Read the model definition and answer for the solid it produces. Units are mm, in the model's axes. A direction names the side the tool comes from. Coordinates: 2 decimals unless noted, no trailing zeros. Order: outer loops, then holes, each group sorted by start corner. A loop starts at its lowest first (then second) coordinate and runs counter-clockwise, first axis right, second up. Notation, with made-up numbers: (63.25, 75.5) -> (104.25, 75.5) arc R16 ccw to (104.25, 104.5) -> close; hole circle Ø11 at (44.25, -31.5). An arc over 180 degrees is marked (long way). Answer as a JSON object with one key per item and string values. Group by question number.
1) A tool of negligible diameter and unlimited length cuts with its end or side. For faces 5 (the flat face through (-65.936, 9, 25)), 6 (the flat face through (-62, 3.499, 28)), 7 (the flat face through (-68, 11.699, 28)), from which of +Z, -Z, +X, -X, +Y, -Y can it reach the whole face along a straight path? Write none if from no direction.
2) Consider L1, parallel to Y at x = -61.75, z = 22; L2, parallel to X at y = 9.75, z = 46.5; L3, parallel to Z at x = -64.75, y = 9. Determine where each line is inside the solid, lowest interval first.
3) Section B-B on x = -60.75 is taken. Determine the outline of the cut face in (y, z).
4) Section A-A on z = 28 is taken. Determine the outline of the cut face in (x, y).
5) Section C-C on y = 10.5 is taken. Determine the outline of the cut face in (x, z).
6) Given pin 1 (6 mm diameter, centred on y = 8.7, z = 28, fed in from +X); pin 2 (1.5 mm diameter, centred on y = 13.5, z = 15.5, fed in from -X); pin 3 (3 mm diameter, centred on y = 10, z = 34.5, fed in from +X), each flat-ended and moving along its own axis, determine where each tip first touches the part or whether it passes through.
7) Section D-D on z = 52.5 is taken. Determine the outline of the cut face in (x, y), and give its area (3 significant figures).
8) Determine the mould class of faces 1 (the flat face through (-65, 9, 0)), 2 (the cylindrical face through (-67.204, 7.355, 30.108)), 3 (the flat face through (-65, 9, 56)), 4 (the flat face through (-68, 5.699, 28)) for opening direction Z: released by +Z, released by -Z, zero draft, split by the parting line, or undercut.
from build123d import *

# Parameters (mm, degrees)
F0_W           = 8
F0_H           = 12
F1_DEPTH       = 56
F2_W           = 5
F2_H           = 10.4
F3_DEPTH       = 56
F5_DEPTH       = 56
F7_D           = 5
F7_DEPTH       = 34
F7_CBORE_D     = 8
F7_CBORE_DEPTH = 1.5
F7_TIP         = 1.5021515476
F8_DEPTH       = 0.5


with BuildPart() as f1:
    # F0 (on Top) → F1 (new body)
    with BuildSketch(Plane.XY):
        with Locations((-63.4363747239, 8.6988127381)):
            Rectangle(F0_W, F0_H)
    extrude(amount=F1_DEPTH)

    # F2 (on face) → F3 (cut)
    with BuildSketch(Plane.XY.offset(56)):
        with Locations((-61.9363747239, 8.6988127381)):
            Rectangle(F2_W, F2_H)
    extrude(amount=-F3_DEPTH, mode=Mode.SUBTRACT)

    # F4 (on face) → F5 (join)
    with BuildSketch(Plane.XY.offset(56)):
        Polygon((-67.4363747239, 5.6988127381), (-67.4363747239, 8.6988127381), (-67.4363747239, 11.6988127381), (-68.4363747239, 11.6988127381), (-68.4363747239, 5.6988127381), align=None)
    extrude(amount=-F5_DEPTH)

    # F7
    with Locations(Plane.YZ.offset(-64.4363747239)):
        with Locations((8.6988127381, 28)):
            CounterBoreHole(F7_D / 2, F7_CBORE_D / 2, F7_CBORE_DEPTH, depth=F7_DEPTH)
            with Locations((0, 0, -(F7_DEPTH + F7_TIP / 2))):  # 118° drill point
                Cone(0, F7_D / 2, F7_TIP, mode=Mode.SUBTRACT)

    # F8 (add): a face of the model
    f8_faces = [f1.faces().sort_by_distance(p)[0] for p in [
        (-64.4363747239, 13.3292374577, 28),
    ]]
    extrude(f8_faces, amount=F8_DEPTH)


solid = f1.part
Worked answers:
{
 "1": {"face 5": "+X", "face 6": "+Z, -Z, +X", "face 7": "+Z, -Z, -X, +Y"},
 "2": {"L1": "y = 2.7 to 3.5, 13.9 to 14.7", "L2": "x = -68.44 to -63.94", "L3": "z = 0 to 24.01, 31.99 to 56"},
 "3": {"outline": "(2.7, 0) -> (3.5, 0) -> (3.5, 56) -> (2.7, 56) -> close; (13.9, 0) -> (14.7, 0) -> (14.7, 56) -> (13.9, 56) -> close"},
 "4": {"outline": "(-68.44, 5.7) -> (-67.44, 5.7) -> (-67.44, 2.7) -> (-59.44, 2.7) -> (-59.44, 3.5) -> (-63.94, 3.5) -> (-63.94, 4.7) -> (-65.94, 4.7) -> (-65.94, 6.2) -> (-68.44, 6.2) -> close; (-68.44, 11.2) -> (-65.94, 11.2) -> (-65.94, 12.7) -> (-63.94, 12.7) -> (-63.94, 13.9) -> (-59.44, 13.9) -> (-59.44, 14.7) -> (-67.44, 14.7) -> (-67.44, 11.7) -> (-68.44, 11.7) -> close"},
 "5": {"outline": "(-68.44, 0) -> (-63.94, 0) -> (-63.94, 24.43) -> (-65.94, 24.43) -> (-65.94, 26.27) -> (-68.44, 26.27) -> close; (-68.44, 29.73) -> (-65.94, 29.73) -> (-65.94, 31.57) -> (-63.94, 31.57) -> (-63.94, 56) -> (-68.44, 56) -> close"},
 "6": {"pin 1": "stops at x = -65.94", "pin 2": "stops at x = -67.44", "pin 3": "stops at x = -63.94"},
 "7": {"outline": "(-68.44, 5.7) -> (-67.44, 5.7) -> (-67.44, 2.7) -> (-59.44, 2.7) -> (-59.44, 3.5) -> (-63.94, 3.5) -> (-63.94, 13.9) -> (-59.44, 13.9) -> (-59.44, 14.7) -> (-67.44, 14.7) -> (-67.44, 11.7) -> (-68.44, 11.7) -> close", "area": "55.2 mm²"},
 "8": {"face 1": "released by -Z", "face 2": "undercut", "face 3": "released by +Z", "face 4": "zero draft"}
}
